Geometry: final body of the model. Coordinates: model frame, mm. A direction names the side the tool comes from. Give positions to 0.01 mm unless a question says otherwise; leave off trailing zeros. Write each loop counter-clockwise with the first axis right and the second up, starting at its lowest first coordinate (ties: lowest second). Pieces come first, ordered by that corner, then holes. Notation, with made-up numbers: (-32, 16) -> (-9, 16) arc R30 ccw to (-9, 41) -> close; hole circle Ø2 at (-29.75, 6). An arc over 180 degrees is marked (long way). Answer in a Markdown table with one row per item. Add a question column.
from build123d import *

# Parameters (mm, degrees)
SKETCH1_W           = 76.2
SKETCH1_H           = 25.4
BOSS_EXTRUDE1_DEPTH = 4.800000052
CUT_EXTRUDE2_DEPTH  = 142.571180171
SKETCH2_W           = 4.500000144
SKETCH2_H           = 16.933333333
CUT_EXTRUDE3_DEPTH  = 142.571180171
SKETCH7_W           = 4.500000144
SKETCH7_H           = 16.933333333
CUT_EXTRUDE4_DEPTH  = 142.571180171
SKETCH8_W           = 0.723333241
SKETCH8_H           = 25.4
CUT_EXTRUDE5_DEPTH  = 142.571180171


with BuildPart() as part:
    # Sketch1 → Boss-Extrude1 (new body)
    with BuildSketch(Plane.XY):
        with Locations((-50.643719603, -97.499415994)):
            Rectangle(SKETCH1_W, SKETCH1_H)
    extrude(amount=BOSS_EXTRUDE1_DEPTH)

    # Sketch6 → Cut-Extrude2 (cut, through all)
    with BuildSketch(Plane.XY.offset(4.800000052)):
        with BuildLine():
            Line((-27.897719629, -110.199415994), (-12.543719603, -110.199415994))
            Line((-12.543719603, -110.199415994), (-12.543719603, -84.799415994))
            Line((-12.543719603, -84.799415994), (-27.897719629, -84.799415994))
            ThreePointArc((-27.897719629, -84.799415994), (-15.197719629, -97.499415994), (-27.897719629, -110.199415994))
        make_face()
    extrude(amount=-CUT_EXTRUDE2_DEPTH, mode=Mode.SUBTRACT)

    # Sketch2 → Cut-Extrude3 (cut, through all)
    with BuildSketch(Plane.XY.offset(4.800000052)):
        with Locations((-24.953719675, -93.266082661)):
            Rectangle(SKETCH2_W, SKETCH2_H)
    extrude(amount=-CUT_EXTRUDE3_DEPTH, mode=Mode.SUBTRACT)

    # Sketch7 → Cut-Extrude4 (cut, through all)
    with BuildSketch(Plane(origin=(0, 0, 0), x_dir=(-1, 0, 0), z_dir=(0, 0, -1))):
        with Locations((77.003719715, -93.266082661)):
            Rectangle(SKETCH7_W, SKETCH7_H)
    extrude(amount=-CUT_EXTRUDE4_DEPTH, mode=Mode.SUBTRACT)

    # Sketch8 → Cut-Extrude5 (cut, through all)
    with BuildSketch(Plane(origin=(0, 0, 0), x_dir=(-1, 0, 0), z_dir=(0, 0, -1))):
        with Locations((88.382052982, -97.499415994)):
            Rectangle(SKETCH8_W, SKETCH8_H)
    extrude(amount=-CUT_EXTRUDE5_DEPTH, mode=Mode.SUBTRACT)


solid = part.part
Q1. Section D-D on y = -103.5. Return loops of the section in (x, z).
Q2. Line query: probe 1 along X at (y, z) = (-86.25, 0.85); probe 2 along X at (y, z) = (-100.5, 0.9); probe 3 along Y at (x, z) = (-77, 2.4). Output: solid intervals per line, ascending. Write a range as from..to.
Q3. Contact query for a flat-ended pin moving along its axis: pin 1 Ø2.5 at (x, z) = (-77.5, 2) entering from +Y. Output: stop coordinate, or through.
Q4. Section B-B on z = 3.1. Return loops of the section in (x, y), and give its area (3 significant figures).
Q5. Pull-direction query (Y, two-part tool) for faces 1 (the cylindrical face through (-15.43, -99.92, 2.43)), 2 (the flat face through (-52, -97, 0)), 3 (the flat face through (-58, -110.199, 2)), 4 (the flat face through (-25, -101.733, 2)); classes: +Y half, -Y half, draft (parallel to the pull), parting line (faces both ways), or undercut.
Q6. Section A-A on y = -89.75. Return loops of the section in (x, z).
Q7. Access query for faces 5 (the flat face through (-88.02, -98, 2)), 6 (the flat face through (-74.754, -93, 2)). Directions: +Z, -Z, +X, -X, +Y, -Y. A direction counts if a zero-diameter tool reaches every point of the face in a straight line with its end or side. Return the directions, or none.
Q8. Section C-C on y = -94.5. Return loops of the section in (x, z), and give its area (3 significant figures).
Checks:
| question | item | result |
|---|---|---|
| 1 | outline | (-88.02, 0) -> (-16.7, 0) -> (-16.7, 4.8) -> (-88.02, 4.8) -> close |
| 2 | probe 1 | -88.02..-79.25, -74.75..-27.2, -22.7..-22 |
| 2 | probe 2 | -88.02..-79.25, -74.75..-27.2, -22.7..-15.56 |
| 2 | probe 3 | -110.2..-101.73 |
| 3 | pin 1 | y = -101.73 |
| 4 | outline | (-88.02, -110.2) -> (-27.9, -110.2) arc R12.7 ccw to (-22.7, -85.91) -> (-22.7, -101.73) -> (-27.2, -101.73) -> (-27.2, -84.82) arc R12.7 ccw to (-27.9, -84.8) -> (-74.75, -84.8) -> (-74.75, -101.73) -> (-79.25, -101.73) -> (-79.25, -84.8) -> (-88.02, -84.8) -> close |
| 4 | area | 1,630 mm^2 |
| 5 | face 1 | parting line |
| 5 | face 2 | draft |
| 5 | face 3 | -Y half |
| 5 | face 4 | +Y half |
| 6 | outline | (-88.02, 0) -> (-79.25, 0) -> (-79.25, 4.8) -> (-88.02, 4.8) -> close; (-74.75, 0) -> (-27.2, 0) -> (-27.2, 4.8) -> (-74.75, 4.8) -> close; (-22.7, 0) -> (-17.84, 0) -> (-17.84, 4.8) -> (-22.7, 4.8) -> close |
| 7 | face 5 | +Z, -Z, -X, +Y, -Y |
| 7 | face 6 | +Z, -Z, +Y |
| 8 | outline | (-88.02, 0) -> (-79.25, 0) -> (-79.25, 4.8) -> (-88.02, 4.8) -> close; (-74.75, 0) -> (-27.2, 0) -> (-27.2, 4.8) -> (-74.75, 4.8) -> close; (-22.7, 0) -> (-15.56, 0) -> (-15.56, 4.8) -> (-22.7, 4.8) -> close |
| 8 | area | 305 mm^2 |
